The listing builds one solid part. Answer for the finished solid, in the listing's coordinates (mm). Face numbers are marked on the shaded views. A direction names the side the tool comes from. Give positions to 0.01 mm unless a question says otherwise; leave off trailing zeros. Write each loop counter-clockwise with the first axis right and the second up, starting at its lowest first coordinate (ties: lowest second). Pieces come first, ordered by that corner, then holes. Notation, with made-up numbers: M 66.25,34.25 L 110.25,34.25 A14 ccw 110.25,59.25 Z; hole C -37.75,4 d4. An arc over 180 degrees is marked long. Answer as a JSON object with one key per item and string values.
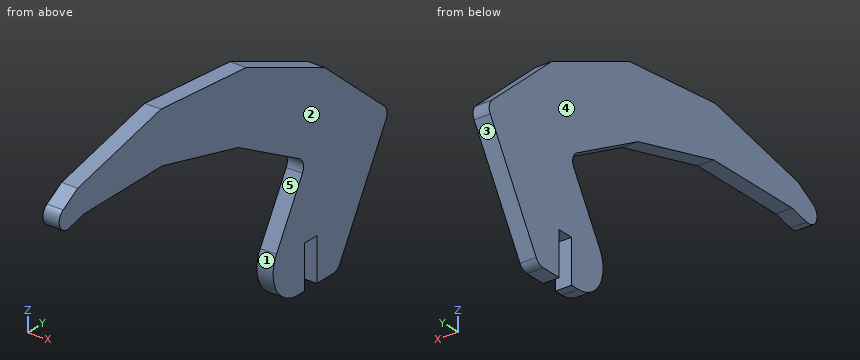
```python
from build123d import *

# Parameters (mm, degrees)
BOSS_EXTRUDE1_DEPTH = 3


with BuildPart() as part:
    # Sketch1 → Boss-Extrude1 (new body)
    with BuildSketch(Plane(origin=(0, 0, 0), x_dir=(0, 0, -1), z_dir=(1, 0, 0))):
        with BuildLine():
            Line((-13.869045208, -53.846884879), (-13.019160894, -57.395119241))
            ThreePointArc((-13.019160894, -57.395119241), (-14.207117004, -59.712178989), (-16.67823792, -58.891467706))
            Line((-16.67823792, -58.891467706), (-18.79288086, -55.373986049))
            Line((-18.79288086, -55.373986049), (-23.446176246, -35.239966644))
            Line((-23.446176246, -35.239966644), (-21.649968985, -14.653428937))
            Line((-21.649968985, -14.653428937), (-13.580084357, 4.370473329))
            Line((-13.580084357, 4.370473329), (-1.081593074, 18.755177998))
            ThreePointArc((-1.081593074, 18.755177998), (0.097807511, 19.415947524), (1.428134813, 19.175465981))
            Line((1.428134813, 19.175465981), (20.650635095, 8.077350269))
            ThreePointArc((20.650635095, 8.077350269), (21.382685902, 7.345299462), (21.650635095, 6.345299462))
            Line((21.650635095, 6.345299462), (21.650635095, 2.5))
            Line((21.650635095, 2.5), (13.650635095, 2.5))
            Line((13.650635095, 2.5), (13.650635095, -0.5))
            Line((13.650635095, -0.5), (21.650635095, -0.5))
            Line((21.650635095, -0.5), (21.650635095, -2.107695155))
            ThreePointArc((21.650635095, -2.107695155), (18.650635095, -7.303847577), (12.650635095, -7.303847577))
            Line((12.650635095, -7.303847577), (1.767371596, -1.020392466))
            ThreePointArc((1.767371596, -1.020392466), (0.230262068, -0.825914438), (-0.984510925, -1.787607726))
            Line((-0.984510925, -1.787607726), (-9.132781883, -16.582681858))
            Line((-9.132781883, -16.582681858), (-13.854695348, -34.915618767))
            Line((-13.854695348, -34.915618767), (-13.869045208, -53.846884879))
        make_face()
    extrude(amount=BOSS_EXTRUDE1_DEPTH)


solid = part.part
```
1. A flat-ended cylindrical pin translates along its axis: pin 1 (1.5 mm diameter, centred on x = 1, y = -51, fed in from +Z). Find the tip coordinate at first contact, or state that the pin passes through.
Verdict:
{"pin 1": "stops at z = 19.98"}
2. A cutting plane is placed at A-A, the plane z = -16. Give the vertices of the cut face in (x, y).
Verdict:
{"outline": "M 0,-8.1 L 3,-8.1 L 3,-0.5 L 0,-0.5 Z; M 0,2.5 L 3,2.5 L 3,10.76 L 0,10.76 Z"}
3. For the marked faces 4 and 5, determine the directions among +Z, -Z, +X, -X, +Y, -Y from which every point of the face is accessible in a straight line to the end or side of a thin tool.
Verdict:
{"face 4": "+Z, -Z, -X, +Y, -Y", "face 5": "+X, -X, -Y"}
4. Consider line 1 along Z through (x, y) = (1.45, -3.5); line 2 along Y through (x, z) = (2.35, -17); line 3 along Y through (x, z) = (0.25, -15). Determine where each line is inside the solid, lowest interval first.
Verdict:
{"line 1": "z = -21.49 to -6.06, 1.93 to 16.92", "line 2": "y = -7.95 to -0.5, 2.5 to 10.19", "line 3": "y = -8.07 to -0.5, 2.5 to 11.34"}
5. A cutting plane is placed at D-D, the plane z = -5.5. Give the vertices of the cut face in (x, y).
Verdict:
{"outline": "M 0,-3.18 L 3,-3.18 L 3,16.82 L 0,16.82 Z"}
6. A cutting plane is placed at C-C, the plane y = -4. Give the vertices of the cut face in (x, z), plus the area to 3 significant figures.
Verdict:
{"outline": "M 0,-21.34 L 3,-21.34 L 3,-6.93 L 0,-6.93 Z; M 0,2.2 L 3,2.2 L 3,17.13 L 0,17.13 Z", "area": "88.0 mm2"}
7. A cutting plane is placed at B-B, the plane x = 1.55. Give the vertices of the cut face in (y, z), plus the area to 3 significant figures.
Verdict:
{"outline": "M -58.89,16.68 A2 ccw -57.4,13.02 L -53.85,13.87 L -34.92,13.85 L -16.58,9.13 L -1.79,0.98 A2 cw -1.02,-1.77 L -7.3,-12.65 A6 ccw -2.11,-21.65 L -0.5,-21.65 L -0.5,-13.65 L 2.5,-13.65 L 2.5,-21.65 L 6.35,-21.65 A2 ccw 8.08,-20.65 L 19.18,-1.43 A2 ccw 18.76,1.08 L 4.37,13.58 L -14.65,21.65 L -35.24,23.45 L -55.37,18.79 Z", "area": "1,160 mm2"}
8. The mould has two halves that part along Z. Classify the marked faces 1, 2 and 3: released by +Z, released by -Z, zero draft, split by the parting line, or undercut.
Verdict:
{"face 1": "undercut", "face 2": "zero draft", "face 3": "released by -Z"}
